from build123d import *

# Parameters (mm, degrees)
SKETCH1_W               = 96
SKETCH1_H               = 21
BOSS_EXTRUDE1_DEPTH     = 3
SKETCH2_W               = 16
SKETCH2_H               = 16
CUT_EXTRUDE3_DEPTH      = 7
CUT_EXTRUDE3_DEPTH_BACK = 7
SKETCH5_W               = 3
SKETCH5_H               = 2.5
SKETCH5_W_2             = 4
BOSS_EXTRUDE5_DEPTH     = 10
SKETCH6_W               = 96
SKETCH6_H               = 21
BOSS_EXTRUDE6_DEPTH     = 2
SKETCH7_R               = 3.5
CUT_EXTRUDE5_DEPTH      = 2
SKETCH9_W               = 114
SKETCH9_H               = 39
BOSS_EXTRUDE7_DEPTH     = 1
SKETCH10_W              = 16
SKETCH10_H              = 16
CUT_EXTRUDE6_DEPTH      = 1


with BuildPart() as part:
    # Sketch1 → Boss-Extrude1 (new body)
    with BuildSketch(Plane(origin=(0, 0, 0), x_dir=(1, 0, 0), z_dir=(0, 1, 0))):
        Rectangle(SKETCH1_W, SKETCH1_H)
    extrude(amount=BOSS_EXTRUDE1_DEPTH)

    # Sketch2 → Cut-Extrude3 (cut, two sides)
    with BuildSketch(Plane(origin=(0, 3, 0), x_dir=(1, 0, 0), z_dir=(0, 1, 0))) as cut_extrude3_sk:
        Rectangle(SKETCH2_W, SKETCH2_H)
        with Locations((-37, 0)):
            Rectangle(SKETCH2_W, SKETCH2_H)
        with Locations((-18.5, 0)):
            Rectangle(SKETCH2_W, SKETCH2_H)
        with Locations((18.5, 0)):
            Rectangle(SKETCH2_W, SKETCH2_H)
        with Locations((37, 0)):
            Rectangle(SKETCH2_W, SKETCH2_H)
    extrude(amount=CUT_EXTRUDE3_DEPTH, mode=Mode.SUBTRACT)
    extrude(cut_extrude3_sk.sketch, amount=-CUT_EXTRUDE3_DEPTH_BACK, mode=Mode.SUBTRACT)

    # Sketch5 → Boss-Extrude5 (add)
    with BuildSketch(Plane(origin=(0, 3, 0), x_dir=(1, 0, 0), z_dir=(0, 1, 0))):
        with Locations((-46.5, 9.25)):
            Rectangle(SKETCH5_W, SKETCH5_H)
        with Locations((-46.5, -9.25)):
            Rectangle(SKETCH5_W, SKETCH5_H)
        with Locations((46.5, 9.25)):
            Rectangle(SKETCH5_W, SKETCH5_H)
        with Locations((46.5, -9.25)):
            Rectangle(SKETCH5_W, SKETCH5_H)
        with Locations((0, 9.25)):
            Rectangle(SKETCH5_W_2, SKETCH5_H)
        with Locations((0, -9.25)):
            Rectangle(SKETCH5_W_2, SKETCH5_H)
    extrude(amount=BOSS_EXTRUDE5_DEPTH)

    # Sketch6 → Boss-Extrude6 (add)
    with BuildSketch(Plane(origin=(0, 13, 0), x_dir=(1, 0, 0), z_dir=(0, 1, 0))):
        Rectangle(SKETCH6_W, SKETCH6_H)
    extrude(amount=BOSS_EXTRUDE6_DEPTH)

    # Sketch7 → Cut-Extrude5 (cut)
    with BuildSketch(Plane(origin=(0, 15, 0), x_dir=(1, 0, 0), z_dir=(0, 1, 0))):
        with Locations((-37, 0)):
            Circle(SKETCH7_R)
        with Locations((-18.5, 0)):
            Circle(SKETCH7_R)
        Circle(SKETCH7_R)
        with Locations((18.5, 0)):
            Circle(SKETCH7_R)
        with Locations((37, 0)):
            Circle(SKETCH7_R)
    extrude(amount=-CUT_EXTRUDE5_DEPTH, mode=Mode.SUBTRACT)

    # Sketch9 → Boss-Extrude7 (add)
    with BuildSketch(Plane.XZ):
        Rectangle(SKETCH9_W, SKETCH9_H)
    extrude(amount=BOSS_EXTRUDE7_DEPTH)

    # Sketch10 → Cut-Extrude6 (cut)
    with BuildSketch(Plane.XZ.offset(1)):
        with Locations((-37, 0)):
            Rectangle(SKETCH10_W, SKETCH10_H)
        with Locations((-18.5, 0)):
            Rectangle(SKETCH10_W, SKETCH10_H)
        Rectangle(SKETCH10_W, SKETCH10_H)
        with Locations((18.5, 0)):
            Rectangle(SKETCH10_W, SKETCH10_H)
        with Locations((37, 0)):
            Rectangle(SKETCH10_W, SKETCH10_H)
    extrude(amount=-CUT_EXTRUDE6_DEPTH, mode=Mode.SUBTRACT)


solid = part.part
Design review of the part built by this model. Coordinates are the model's own, in mm. A direction names the side the tool comes from. Give positions to 0.01 mm unless a question says otherwise; leave off trailing zeros. Write each loop counter-clockwise with the first axis right and the second up, starting at its lowest first coordinate (ties: lowest second). Pieces come first, ordered by that corner, then holes. Notation, with made-up numbers: M 27.25,20.5 L 73.25,20.5 A30 cw 73.25,46.5 Z; hole C 73.5,5 d11. An arc over 180 degrees is marked long. Return JSON: item names as keys, results as strings. Group by question number.
Item 1: Take a section at C-C (y = 7.5). Give the boundary of the cut face in (x, z), plus the area to 3 significant figures.
Item 2: Wall thickness on line 1 along X through (y, z) = (14.2, 0); line 2 along X through (y, z) = (2.5, 0); line 3 along X through (y, z) = (4.25, -9): over which ranges is each line inside the solid? List them lowest first.
Item 3: Tool access review of faces 4 (the cylindrical face through (21.84, 14.01, -1.05)), 5 (the flat face through (46, 8, 8)), 6 (the flat face through (-45, 8, 9)), 7 (the flat face through (-10.5, 1, 0)): name each direction out of +Z, -Z, +X, -X, +Y, -Y from which nothing blocks a thin tool from reaching the whole face with its end or side.
Item 4: Take a section at D-D (x = -37). Give the boundary of the cut face in (y, z), plus the area to 3 significant figures.
Item 5: Clearance check with flat-ended pins moving along their axes: pin 1 Ø5 at (y, z) = (6.5, -11) entering from +X; pin 2 Ø2 at (x, y) = (-37, 1.5) entering from -Z; pin 3 Ø6 at (y, z) = (2.5, -7.5) entering from +X; pin 4 Ø1.2 at (y, z) = (2, -3) entering from -X. State where each tip first meets the part, or that it passes through.
Item 6: Take a section at B-B (x = -4.5). Give the boundary of the cut face in (y, z).
Item 7: Take a section at A-A (z = -5). Count the separate pieces of the cut face and the enclosed holes in it, plus the area to 3 significant figures.
Item 8: The part is to be moulded in two halves that separate along X. For faces 1 (the flat face through (-48, 2, 0)), 2 (the flat face through (-47, 8, 8)), 3 (the flat face through (45, 8, -9)), say which applies: pulls with the +X half, pulls with the -X half, needs draft (parallel to the pull), parting line crosses it, or undercut.
Return value:
{
 "1": {"outline": "M -48,-10.5 L -45,-10.5 L -45,-8 L -48,-8 Z; M -48,8 L -45,8 L -45,10.5 L -48,10.5 Z; M -2,-10.5 L 2,-10.5 L 2,-8 L -2,-8 Z; M -2,8 L 2,8 L 2,10.5 L -2,10.5 Z; M 45,-10.5 L 48,-10.5 L 48,-8 L 45,-8 Z; M 45,8 L 48,8 L 48,10.5 L 45,10.5 Z", "area": "50.0 mm2"},
 "2": {"line 1": "x = -48 to -40.5, -33.5 to -22, -15 to -3.5, 3.5 to 15, 22 to 33.5, 40.5 to 48", "line 2": "x = -48 to -45, -29 to -26.5, -10.5 to -8, 8 to 10.5, 26.5 to 29, 45 to 48", "line 3": "x = -48 to -45, -2 to 2, 45 to 48"},
 "3": {"face 4": "+Y, -Y", "face 5": "+X, -X", "face 6": "+Z, -Z", "face 7": "-Y"},
 "4": {"outline": "M -1,-19.5 L 0,-19.5 L 0,-10.5 L 3,-10.5 L 3,-8 L -1,-8 Z; M -1,8 L 3,8 L 3,10.5 L 0,10.5 L 0,19.5 L -1,19.5 Z; M 13,-10.5 L 15,-10.5 L 15,-3.5 L 13,-3.5 Z; M 13,3.5 L 15,3.5 L 15,10.5 L 13,10.5 Z", "area": "66.0 mm2"},
 "5": {"pin 1": "stops at x = 48", "pin 2": "stops at z = -10.5", "pin 3": "stops at x = 57", "pin 4": "stops at x = -48"},
 "6": {"outline": "M -1,-19.5 L 0,-19.5 L 0,-10.5 L 3,-10.5 L 3,-8 L -1,-8 Z; M -1,8 L 3,8 L 3,10.5 L 0,10.5 L 0,19.5 L -1,19.5 Z; M 13,-10.5 L 15,-10.5 L 15,10.5 L 13,10.5 Z"},
 "7": {"separate pieces": "7", "enclosed holes": "0", "area": "274 mm2"},
 "8": {"face 1": "pulls with the -X half", "face 2": "needs draft", "face 3": "undercut"}
}
